Part model, mm, in its own coordinate system. Round coordinates to 2 decimals unless told otherwise and drop trailing zeros. Write each loop counter-clockwise with the first axis right and the second up, starting at its lowest first coordinate (ties: lowest second). Pieces come first, ordered by that corner, then holes. Notation, with made-up numbers: M 84,-16 L 119,-16 A18 ccw 119,8 Z; hole C 79,5.5 d8. An arc over 180 degrees is marked long. Answer as a JSON object with one key per item and string values. Group by question number.
1. Drop flat-ended pins along their axis: pin 1 (3 mm diameter, centred on x = 12.5, z = 6, fed in from +Y); pin 2 (3 mm diameter, centred on x = 96.5, y = 10.5, fed in from +Z); pin 3 (1 mm diameter, centred on x = 11.5, z = 7, fed in from -Y). Give the stop position or say it passes through.
2. Band-saw the part on B-B, the plane x = 15. Write the cut outline in (y, z), plus the area to 3 significant figures.
3. Drill centre lines: line 1 (Y direction, x = 95, z = 2.2); line 2 (Y direction, x = 95, z = 4.45); line 3 (X direction, y = 7.5, z = 3.75). Where is each one in solid material? Low to high. Write a range as from..to.
4. Band-saw the part on C-C, the plane y = 8. Write the cut outline in (x, z), plus the area to 3 significant figures.
5. Band-saw the part on A-A, the plane z = 5. Write the cut outline in (x, y), plus the area to 3 significant figures.
6. Band-saw the part on D-D, the plane x = 58.5. Write the cut outline in (y, z), plus the area to 3 significant figures.
from build123d import *

# Parameters (mm, degrees)
F0_W     = 110
F0_H     = 20
F0_R     = 3
F1_DEPTH = 3
F2_R     = 3.25
F3_DEPTH = 5


with BuildPart() as f1:
    # F0 (on Top) → F1 (new body)
    with BuildSketch(Plane.XY):
        with Locations((55, 10)):
            Rectangle(F0_W, F0_H)
        with Locations((15, 10)):
            Circle(F0_R, mode=Mode.SUBTRACT)
        with Locations((95, 10)):
            Circle(F0_R, mode=Mode.SUBTRACT)
    extrude(amount=F1_DEPTH)

    # F2 (on face) → F3 (join)
    with BuildSketch(Plane.XY.offset(3)):
        Polygon((17.886751, 5), (20.773503, 10), (17.886751, 15), (12.113249, 15), (9.226497, 10), (12.113249, 5), align=None)
        with Locations((15, 10)):
            Circle(F2_R, mode=Mode.SUBTRACT)
        Polygon((97.886751, 5), (100.773503, 10), (97.886751, 15), (92.113249, 15), (89.226497, 10), (92.113249, 5), align=None)
        with Locations((95, 10)):
            Circle(F2_R, mode=Mode.SUBTRACT)
    extrude(amount=F3_DEPTH)


solid = f1.part
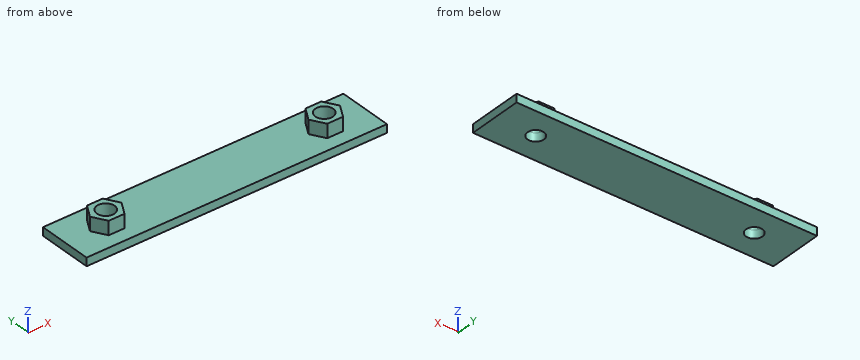
Worked answers:
{
 "1": {"pin 1": "stops at y = 15", "pin 2": "stops at z = 3", "pin 3": "stops at y = 5.2"},
 "2": {"outline": "M 0,0 L 7,0 L 7,3 L 6.75,3 L 6.75,8 L 5,8 L 5,3 L 0,3 Z; M 13,0 L 20,0 L 20,3 L 15,3 L 15,8 L 13.25,8 L 13.25,3 L 13,3 Z", "area": "59.5 mm^2"},
 "3": {"line 1": "y = 0..7, 13..20", "line 2": "y = 5..6.75, 13.25..15", "line 3": "x = 10.67..12.92, 17.08..19.33, 90.67..92.92, 97.08..99.33"},
 "4": {"outline": "M 0,0 L 12.76,0 L 12.76,3 L 12.44,3 L 12.44,8 L 10.38,8 L 10.38,3 L 0,3 Z; M 17.24,0 L 92.76,0 L 92.76,3 L 92.44,3 L 92.44,8 L 90.38,8 L 90.38,3 L 19.62,3 L 19.62,8 L 17.56,8 L 17.56,3 L 17.24,3 Z; M 97.24,0 L 110,0 L 110,3 L 99.62,3 L 99.62,8 L 97.56,8 L 97.56,3 L 97.24,3 Z", "area": "344 mm^2"},
 "5": {"outline": "M 9.23,10 L 12.11,5 L 17.89,5 L 20.77,10 L 17.89,15 L 12.11,15 Z; M 89.23,10 L 92.11,5 L 97.89,5 L 100.77,10 L 97.89,15 L 92.11,15 Z; hole C 15,10 d6.5; hole C 95,10 d6.5", "area": "107 mm^2"},
 "6": {"outline": "M 0,0 L 20,0 L 20,3 L 0,3 Z", "area": "60.0 mm^2"}
}
